Build history of the part. All positions in model axes, mm. A direction names the side the tool comes from. Coordinates: 2 decimals unless noted, no trailing zeros. Order: outer loops, then holes, each group sorted by start corner. A loop starts at its lowest first (then second) coordinate and runs counter-clockwise, first axis right, second up. Notation, with made-up numbers: M 70.5,25 L 90.5,25 A10 cw 90.5,32 Z; hole C 13,12 d4. An arc over 180 degrees is marked long. Use a Markdown table: item, result. Add a question column.
from build123d import *

# Parameters (mm, degrees)
BOSS_EXTRUDE1_DEPTH = 25.4
SKETCH3_W           = 13.97
SKETCH3_H           = 7.62
CUT_EXTRUDE1_DEPTH  = 78.261522765
SKETCH4_W           = 31.117855917
SKETCH4_H           = 3.175
BOSS_EXTRUDE2_DEPTH = 55.88


with BuildPart() as part:
    # Sketch2 → Boss-Extrude1 (new body)
    with BuildSketch(Plane.XY):
        Polygon((0, 0), (0.632144083, 62.23), (3.807144083, 62.23), (3.807144083, 6.35), (34.925, 6.35), (34.925, 62.23), (38.1, 62.23), (38.1, 0), align=None)
    extrude(amount=BOSS_EXTRUDE1_DEPTH)

    # Sketch3 → Cut-Extrude1 (cut, through all)
    with BuildSketch(Plane(origin=(38.1, 0, 0), x_dir=(0, 0, -1), z_dir=(1, 0, 0))):
        with Locations((-12.7, 11.43)):
            Rectangle(SKETCH3_W, SKETCH3_H)
    extrude(amount=-CUT_EXTRUDE1_DEPTH, mode=Mode.SUBTRACT)

    # Sketch4 → Boss-Extrude2 (add)
    with BuildSketch(Plane(origin=(0, 6.35, 0), x_dir=(1, 0, 0), z_dir=(0, 1, 0))):
        with Locations((19.366072042, -1.5875)):
            Rectangle(SKETCH4_W, SKETCH4_H)
        with Locations((19.366072042, -23.8125)):
            Rectangle(SKETCH4_W, SKETCH4_H)
    extrude(amount=BOSS_EXTRUDE2_DEPTH)


solid = part.part
(1) Slice it at A-A on z = 8.5. Give the cut face in (x, y) (3 decimals).
(2) Which spindle directions (+Z, -Z, +X, -X, +Y, -Y) get a long thin tool onto all of the face, cutting with end or side? Do faces 5 (the flat face through (19, 31, 0)), 6 (the flat face through (2, 15.24, 13)), 7 (the flat face through (34.925, 34, 13)). Say none if no direction does.
(3) Drop flat-ended pins along their axis: P1, Ø2, axis at x = 20.5, z = 20.5, coming from the +Y side; P2, Ø3, axis at y = 18, z = 7.5, coming from the -X side. Give the stop position or say it passes through.
(4) Mould opens along Y. For faces 1 (the flat face through (19, 34, 3.175)), 2 (the flat face through (37, 11, 5.715)), 3 (the flat face through (37, 15.24, 13)), 4 (the flat face through (19, 6.35, 13)) say: released by +Y, released by -Y, zero draft, split by the parting line, or undercut.
(5) Drill centre lines: line 1 along Y through (x, z) = (35, 14.25); line 2 along Z through (x, y) = (28, 25) (3 decimals); line 3 along Y through (x, z) = (11, 8.5). Where is each one in solid material? Low to high. Write a range as from..to.
(6) Slice it at B-B on y = 13.5. Give the cut face in (x, z) (3 decimals), and give its area (3 significant figures).
(7) Slice it at C-C on x = 16. Give the cut face in (y, z) (3 decimals), and give its area (3 significant figures).
(8) Slice it at D-D on y = 35.5. Give the cut face in (x, z) (3 decimals).
Solutions:
| question | item | result |
|---|---|---|
| 1 | outline | M 0,0 L 38.1,0 L 38.1,7.62 L 34.925,7.62 L 34.925,6.35 L 3.807,6.35 L 3.807,7.62 L 0.077,7.62 Z; M 0.155,15.24 L 3.807,15.24 L 3.807,62.23 L 0.632,62.23 Z; M 34.925,15.24 L 38.1,15.24 L 38.1,62.23 L 34.925,62.23 Z |
| 2 | face 5 | -Z, +X, -X, +Y, -Y |
| 2 | face 6 | +X, -X |
| 2 | face 7 | +Y |
| 3 | P1 | y = 6.35 |
| 3 | P2 | x = 0.17 |
| 4 | face 1 | zero draft |
| 4 | face 2 | undercut |
| 4 | face 3 | undercut |
| 4 | face 4 | released by +Y |
| 5 | line 1 | 0..7.62, 15.24..62.23 |
| 5 | line 2 | 0..3.175, 22.225..25.4 |
| 5 | line 3 | 0..6.35 |
| 6 | outline | M 0.137,0 L 38.1,0 L 38.1,5.715 L 34.925,5.715 L 34.925,3.175 L 3.807,3.175 L 3.807,5.715 L 0.137,5.715 Z; M 0.137,19.685 L 3.807,19.685 L 3.807,22.225 L 34.925,22.225 L 34.925,19.685 L 38.1,19.685 L 38.1,25.4 L 0.137,25.4 Z |
| 6 | area | 276 mm² |
| 7 | outline | M 0,0 L 62.23,0 L 62.23,3.175 L 6.35,3.175 L 6.35,22.225 L 62.23,22.225 L 62.23,25.4 L 0,25.4 Z |
| 7 | area | 516 mm² |
| 8 | outline | M 0.361,0 L 38.1,0 L 38.1,25.4 L 0.361,25.4 Z; hole M 3.807,3.175 L 34.925,3.175 L 34.925,22.225 L 3.807,22.225 Z |
